```python
from build123d import *

# Parameters (mm, degrees)
F0_R     = 55
F1_DEPTH = 50
F2_W     = 20
F2_H     = 20
F3_DEPTH = 30
F3_TAPER = -15
F5_DEPTH = 100


with BuildPart() as f1:
    # F0 (on Top) → F1 (new body)
    with BuildSketch(Plane.XY):
        Circle(F0_R)
    extrude(amount=F1_DEPTH)

    # F2 (on face) → F3 (join)
    with BuildSketch(Plane.XY.offset(50)):
        with Locations((-10, -10)):
            Rectangle(F2_W, F2_H)
    extrude(amount=F3_DEPTH, taper=F3_TAPER)

    # F4 (on face) → F5 (cut)
    with BuildSketch(Plane.XY.offset(80)):
        Polygon((0.0648668621, -4.1890464078), (-10, 1.6219071844), (-20.0648668621, -4.1890464078), (-20.0648668621, -15.8109535922), (-10, -21.6219071844), (0.0648668621, -15.8109535922), align=None)
    extrude(amount=-F5_DEPTH, mode=Mode.SUBTRACT)


solid = f1.part
```
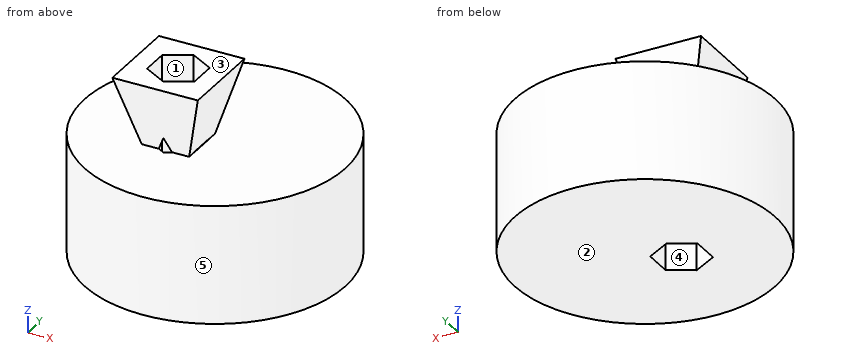
Design review of the part built by this model. Coordinates are the model's own, in mm. Face numbers are marked on the shaded views. A direction names the side the tool comes from. Coordinates: 2 decimals unless noted, no trailing zeros. Order: outer loops, then holes, each group sorted by start corner. A loop starts at its lowest first (then second) coordinate and runs counter-clockwise, first axis right, second up. Notation, with made-up numbers: (60, 8.5) -> (115, 8.5) arc R22 ccw to (115, 23.5) -> close; hole circle Ø6 at (-35.5, 17.25). An arc over 180 degrees is marked (long way). One line per item, written item: value. Start each with the question number.
Q1. Insertion check: pin 1 Ø1.5 at (y, z) = (20, 48) entering from +X; pin 2 Ø5 at (x, z) = (37, 30.5) entering from +Y; pin 3 Ø4 at (x, z) = (-9.5, 11) entering from +Y; pin 4 Ø12 at (x, y) = (-28.5, 14) entering from -Z. Each pin has a flat end and moves straight along its axis. Give the tip position at first contact, or say it passes through.
Q2. For probe 1 along Z at (x, y) = (25, 23); probe 2 along X at (y, z) = (-17.5, 18.5); probe 3 along Y at (x, z) = (-9, 28), list the stretches that pass through material, from the lowest coordinate up.
Q3. Take a section at D-D, the plane y = 28. State the section outline as (x, z) points, then the cut area to 3 significant figures.
Q4. Tool access review of the marked faces 1 and 2: name each direction out of +Z, -Z, +X, -X, +Y, -Y from which nothing blocks a thin tool from reaching the whole face with its end or side.
Q5. Take a section at C-C, the plane x = 25.5. State the section outline as (y, z) points, then the cut area to 3 significant figures.
Q6. Take a section at A-A, the plane z = 46.5. State the section outline as (x, y) points, then the cut area to 3 significant figures.
Q7. Take a section at B-B, the plane y = -14. Give the number of separate pieces and of enclosed holes in the cut face, then the cut area to 3 significant figures.
Q8. Mouldability with a two-part tool opening along Y and no side actions: class the marked faces 3, 4 and 5 as pulls with the +Y half, pulls with the -Y half, needs draft (parallel to the pull), parting line crosses it, or undercut.
Values follow:
1. pin 1: stops at x = 51.52
1. pin 2: stops at y = 42.83
1. pin 3: stops at y = 54.49
1. pin 4: stops at z = 0
2. probe 1: z = 0 to 50
2. probe 2: x = -52.14 to -17.14, -2.86 to 52.14
2. probe 3: y = -54.26 to -21.04, 1.04 to 54.26
3. outline: (-47.34, 0) -> (47.34, 0) -> (47.34, 50) -> (-47.34, 50) -> close
3. area: 4,730 mm2
4. face 1: +Z, -Z
4. face 2: -Z, +X, -X, +Y, -Y
5. outline: (-48.73, 0) -> (48.73, 0) -> (48.73, 50) -> (-48.73, 50) -> close
5. area: 4,870 mm2
6. outline: circle Ø110 at (0, 0); hole (-20.06, -15.81) -> (-10, -21.62) -> (0.06, -15.81) -> (0.06, -4.19) -> (-10, 1.62) -> (-20.06, -4.19) -> close
6. area: 9,150 mm2
7. separate pieces: 4
7. enclosed holes: 0
7. area: 4,550 mm2
8. face 3: needs draft
8. face 4: undercut
8. face 5: parting line crosses it
